Answer from the drawing. Dimensions are ordinates in mm from the lowest x, y and z of the part. A direction names the side the tool comes from. Coordinates: 2 decimals unless noted, no trailing zeros. Write each loop counter-clockwise with the first axis right and the second up, starting at its lowest first coordinate (ties: lowest second). Pieces come first, ordered by that corner, then holes.
(1) Straight lines are drawn through the part: line 1 (Y direction, x = 51, z = 16); line 2 (Z direction, x = 31.5, y = 14.75); line 3 (X direction, y = 14.5, z = 39.5). For each, find the intervals that lie inside material, in ascending order.
(2) The part is cut by section C-C on z = 47.5. Determine the outline of the cut face in (x, y).
(3) Given P1, Ø4.5, axis at y = 8.5, z = 16, coming from the +X side; P2, Ø6, axis at x = 6, y = 8.5, coming from the +Z side; P3, Ø8.5, axis at y = 10.5, z = 36.5, coming from the -X side, each flat-ended and moving along its own axis, determine where each tip first touches the part or whether it passes through.
(4) The part is cut by section B-B on y = 7. Determine the outline of the cut face in (x, z), plus the area to 3 significant figures.
(5) The part is cut by section D-D on y = 14.5. Determine the outline of the cut face in (x, z).
(6) The part is cut by section A-A on x = 6. Determine the outline of the cut face in (y, z).
(7) Which of the six approach directions +Z, -Z, +X, -X, +Y, -Y give full straight-line access (tool end or side, diameter ignored) to the marked faces 1 and 2?
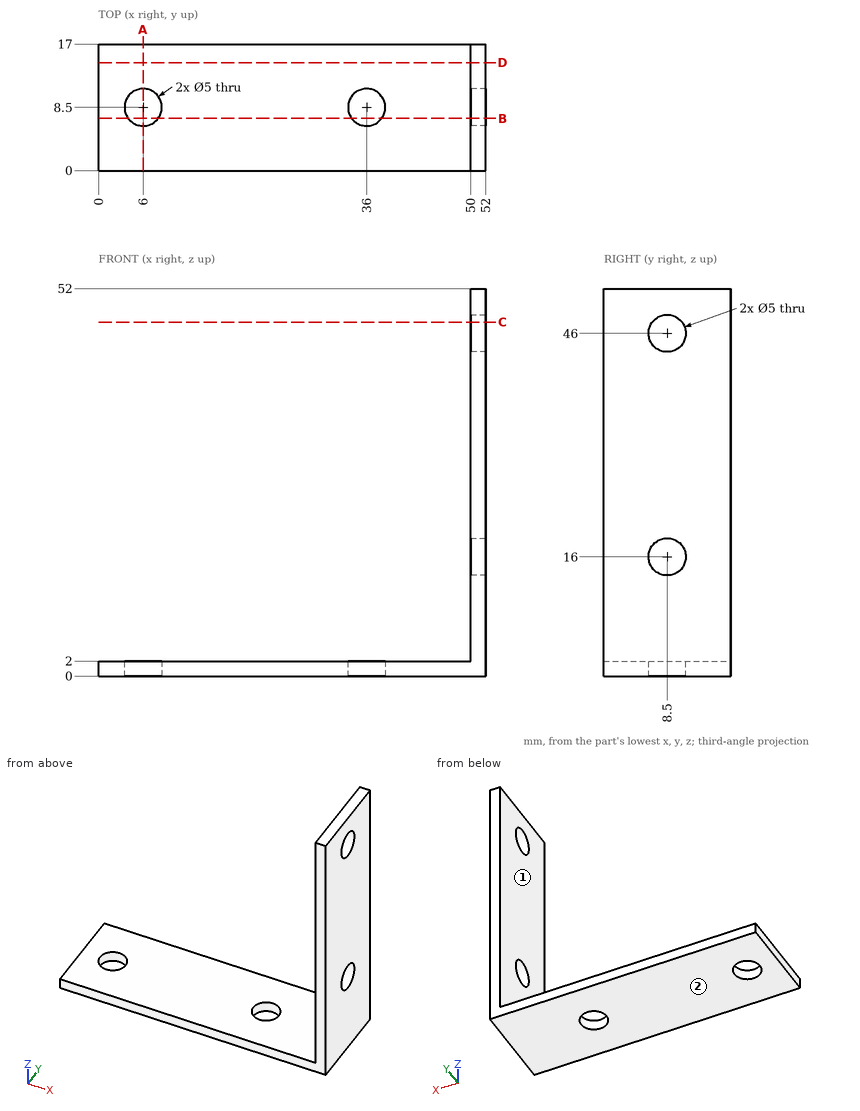
Model answer:
1. line 1: y = 0 to 6, 11 to 17
1. line 2: z = 0 to 2
1. line 3: x = 50 to 52
2. outline: (50, 0) - (52, 0) - (52, 6.5) - (50, 6.5) - close; (50, 10.5) - (52, 10.5) - (52, 17) - (50, 17) - close
3. P1: passes through
3. P2: stops at z = 2
3. P3: stops at x = 50
4. outline: (0, 0) - (4, 0) - (4, 2) - (0, 2) - close; (8, 0) - (34, 0) - (34, 2) - (8, 2) - close; (38, 0) - (52, 0) - (52, 14) - (50, 14) - (50, 2) - (38, 2) - close; (50, 18) - (52, 18) - (52, 44) - (50, 44) - close; (50, 48) - (52, 48) - (52, 52) - (50, 52) - close
4. area: 172 mm2
5. outline: (0, 0) - (52, 0) - (52, 52) - (50, 52) - (50, 2) - (0, 2) - close
6. outline: (0, 0) - (6, 0) - (6, 2) - (0, 2) - close; (11, 0) - (17, 0) - (17, 2) - (11, 2) - close
7. face 1: +Z, -X, +Y, -Y
7. face 2: -Z, +X, -X, +Y, -Y
